Can you work these out from the drawing? Everything is in mm from the part's minimum corner. A direction names the side the tool comes from. Give positions to 0.01 mm unless a question says otherwise; leave off trailing zeros. Order: outer loops, then holes, each group sorted by start corner. A loop starts at its lowest first (then second) coordinate and runs counter-clockwise, first axis right, second up. Notation, with made-up numbers: (48, 63) - (91, 63) arc R26 cw to (91, 99) - close; hole circle Ø4 at (59, 4). An arc over 180 degrees is marked (long way). One line per question, with ' | ' between items.
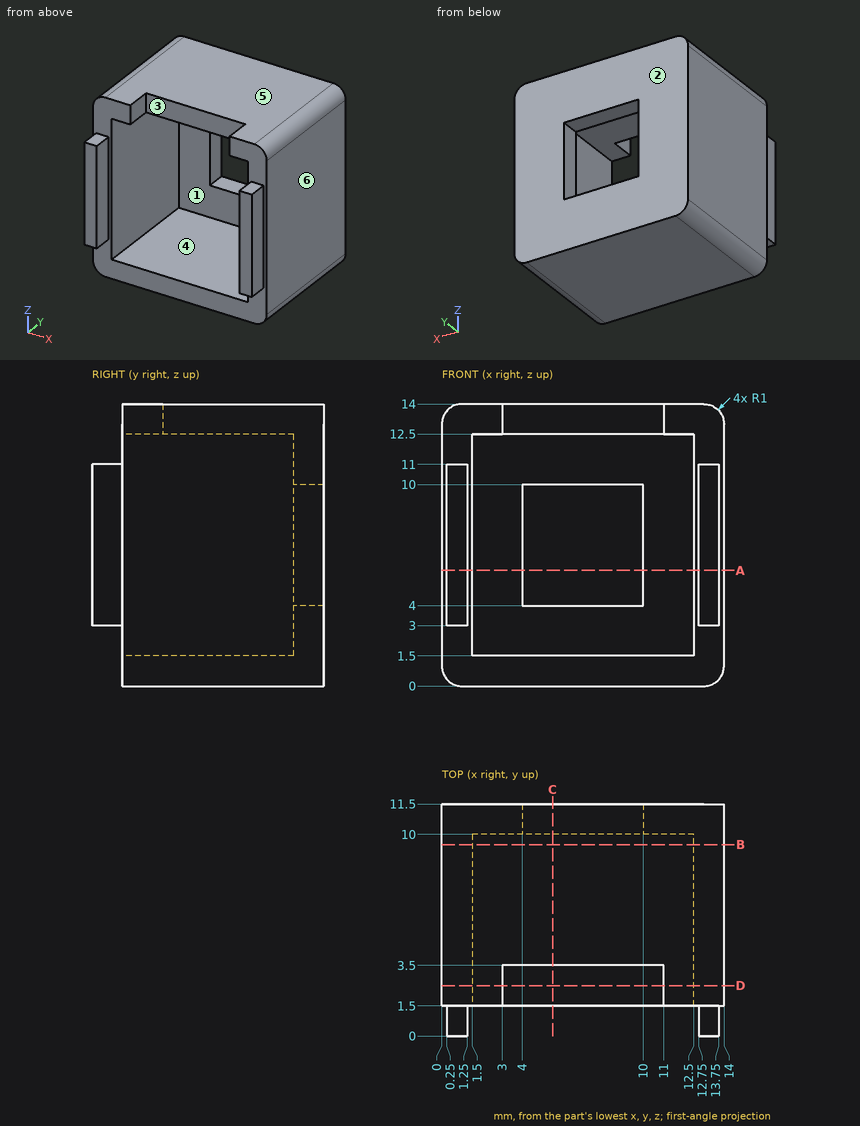
(1) On a 3-axis mill with a long thin cutter (end or side, diameter ignored), from which of +Z, -Z, +X, -X, +Y, -Y can I reach the whole of each face in a straight line? I mean the marked faces 1, 2 and 3. Say none if no direction works.
Answer below:
face 1: -Y | face 2: +Z, -Z, +X, -X, +Y | face 3: +Z, -Y
(2) Imagine slicing it at D-D (y = 2.5). List the corners of the cut face in (x, z) for me, and give its area (3 significant figures).
Answer below:
outline: (0, 1) arc R1 ccw to (1, 0) - (13, 0) arc R1 ccw to (14, 1) - (14, 13) arc R1 ccw to (13, 14) - (11, 14) - (11, 12.5) - (12.5, 12.5) - (12.5, 1.5) - (1.5, 1.5) - (1.5, 12.5) - (3, 12.5) - (3, 14) - (1, 14) arc R1 ccw to (0, 13) - close | area: 62.1 mm^2
(3) If we mould it in two halves opening along X, with no side actions, what happens to the marked faces 4, 5 and 6? For each: released by +X, released by -X, zero draft, split by the parting line, or undercut.
Answer below:
face 4: undercut | face 5: zero draft | face 6: released by +X
(4) Imagine slicing it at B-B (y = 9.5). List the corners of the cut face in (x, z) for me, and give its area (3 significant figures).
Answer below:
outline: (0, 1) arc R1 ccw to (1, 0) - (13, 0) arc R1 ccw to (14, 1) - (14, 13) arc R1 ccw to (13, 14) - (1, 14) arc R1 ccw to (0, 13) - close; hole (1.5, 1.5) - (12.5, 1.5) - (12.5, 12.5) - (1.5, 12.5) - close | area: 74.1 mm^2
(5) If I drill on line 1 (Z direction, x = 4.75, y = 10.5); line 2 (X direction, y = 2.5, z = 3.25), over which ranges is the centre line in solid material (lowest first)?
Answer below:
line 1: 0 to 4, 10 to 14 | line 2: 0 to 1.5, 12.5 to 14
(6) Imagine slicing it at A-A (z = 5.75). List the corners of the cut face in (x, y) for me, and give its area (3 significant figures).
Answer below:
outline: (0, 1.5) - (0.25, 1.5) - (0.25, 0) - (1.25, 0) - (1.25, 1.5) - (1.5, 1.5) - (1.5, 10) - (4, 10) - (4, 11.5) - (0, 11.5) - close; (10, 10) - (12.5, 10) - (12.5, 1.5) - (12.75, 1.5) - (12.75, 0) - (13.75, 0) - (13.75, 1.5) - (14, 1.5) - (14, 11.5) - (10, 11.5) - close | area: 40.5 mm^2
(7) Imagine slicing it at C-C (x = 5.5). List the corners of the cut face in (y, z) for me, and give its area (3 significant figures).
Answer below:
outline: (1.5, 0) - (11.5, 0) - (11.5, 4) - (10, 4) - (10, 1.5) - (1.5, 1.5) - close; (3.5, 12.5) - (10, 12.5) - (10, 10) - (11.5, 10) - (11.5, 14) - (3.5, 14) - close | area: 34.5 mm^2
(8) Will these pins go through, and if not, where does the flat tip stop? pin 1 (1 mm diameter, centred on x = 5.5, z = 6, fed in from -Y); pin 2 (4 mm diameter, centred on x = 5, z = 9, fed in from -Y); pin 3 (1.2 mm diameter, centred on x = 7.5, z = 13, fed in from -Y); pin 4 (0.5 mm diameter, centred on x = 1, y = 1, fed in from +Z).
Answer below:
pin 1: through | pin 2: y = 10 | pin 3: y = 3.5 | pin 4: z = 11
